Could you check a few things on this model? Use its own coordinates, in mm. A direction names the side the tool comes from. Coordinates: 2 decimals unless noted, no trailing zeros. Loops run counter-clockwise (first coordinate to the right, second up) from the corner with the lowest first, then second, coordinate; pieces in that order, holes last. Notation, with made-up numbers: (76.25, 14.25) - (100.25, 14.25) arc R13 ccw to (100.25, 18.25) - close; hole circle Ø2 at (83, 29.25). An arc over 180 degrees is marked (long way). One line per question, with ' | ' between items. Start each with the question number.
1. I want a section at B-B, the plane z = 3. Count the separate pieces of the cut face and the enclosed holes in it, then the cut area to 3 significant figures.
2. I want a section at A-A, the plane x = 246.5. Write out the boundary of the cut face in (y, z).
3. We'd pull the mould along Y, two halves only. Please class faces 1 (the flat face through (247, 422, 0)), 2 (the flat face through (265.41, 446.46, 3.7)), 3 (the cylindrical face through (303.067, 434.436, 3.698)), 4 (the flat face through (231.455, 384.982, 3.698)): pulls with the +Y half, pulls with the -Y half, needs draft (parallel to the pull), parting line crosses it, or undercut.
4. Please list where these lines run through material, in increasing order: L1, parallel to Y at x = 241.5, z = 1.25; L2, parallel to Y at x = 276.5, z = 6; L3, parallel to X at y = 426.5, z = 3.25. Write a range as [from, to].
5. I'm going to push flat-ended pins straight in: P1, Ø4, axis at y = 408.5, z = 6, coming from the -X side; P2, Ø4, axis at x = 204.5, y = 400, coming from the +Z side; P3, Ø2, axis at y = 389.5, z = 4.5, coming from the -X side; P4, Ø3, axis at x = 252.5, z = 4, coming from the -Y side. Where does each tip first touch, or does it pass through?
6. Which directions (+Z, -Z, +X, -X, +Y, -Y) give clear straight access to the entire face, cutting with the end or side of a thin tool? Please do faces 5 (the cylindrical face through (279.122, 439.862, 3.698)), 6 (the flat face through (203.159, 445.655, 3.698)).
from build123d import *

# Parameters (mm, degrees)
SKETCH1_R           = 13.83528528
SKETCH1_R_2         = 7.213103978
SKETCH1_R_3         = 7.235591107
SKETCH1_R_4         = 7.205059389
SKETCH1_R_5         = 3.002887994
SKETCH1_R_6         = 3.006464833
SKETCH1_R_7         = 3.009410698
SKETCH1_R_8         = 3.002883417
SKETCH1_R_9         = 3.011320737
BOSS_EXTRUDE3_DEPTH = 10
SCALE6_SCALE        = 0.75


with BuildPart() as part:
    # Sketch1 → Boss-Extrude3 (new body)
    with BuildSketch(Plane.XY):
        with BuildLine():
            Line((388.937137401, 591.801924948), (317.8384, 598.8518))
            Line((317.8384, 598.8518), (286.3759, 593.1514))
            Line((286.3759, 593.1514), (254.9413, 595.2929))
            add(Edge.make_bspline(
                [(254.9413, 595.2929), (249.749, 589.6403), (247.5763, 576.1381), (246.6964, 565.0014)],
                knots=[0.333333333, 0.333333333, 0.333333333, 0.333333333, 0.375, 0.375, 0.375, 0.375], degree=3))
            add(Edge.make_bspline(
                [(246.6964, 565.0014), (246.2536, 559.3969), (253.8266, 545.9237), (260.2361, 536.2788)],
                knots=[0.375, 0.375, 0.375, 0.375, 0.416666667, 0.416666667, 0.416666667, 0.416666667], degree=3))
            add(Edge.make_bspline(
                [(260.2361, 536.2788), (261.9315, 533.7276), (265.3965, 528.2241), (269.3831, 526.0001)],
                knots=[0.416666667, 0.416666667, 0.416666667, 0.416666667, 0.458333333, 0.458333333, 0.458333333, 0.458333333], degree=3))
            add(Edge.make_bspline(
                [(269.3831, 526.0001), (274.7125, 523.027), (280.9349, 523.6791), (284.7215, 523.5997)],
                knots=[0.458333333, 0.458333333, 0.458333333, 0.458333333, 0.5, 0.5, 0.5, 0.5], degree=3))
            Line((284.7215, 523.5997), (294.3118, 523.3986))
            add(Edge.make_bspline(
                [(294.3118, 523.3986), (298.656, 523.1896), (301.8697, 521.53), (304.1649, 518.6915)],
                knots=[0.541666667, 0.541666667, 0.541666667, 0.541666667, 0.583333333, 0.583333333, 0.583333333, 0.583333333], degree=3))
            Line((304.1649, 518.6915), (313.1736, 507.7735))
            add(Edge.make_bspline(
                [(313.1736, 507.7735), (316.1604, 504.7059), (319.8516, 502.9821), (324.4499, 502.9891)],
                knots=[0.625, 0.625, 0.625, 0.625, 0.666666667, 0.666666667, 0.666666667, 0.666666667], degree=3))
            Line((324.4499, 502.9891), (362.1482, 502.591))
            add(Edge.make_bspline(
                [(362.1482, 502.591), (370.3987, 506.5747), (383.2456, 509.8601), (391.8953, 515.4769)],
                knots=[0.708333333, 0.708333333, 0.708333333, 0.708333333, 0.75, 0.75, 0.75, 0.75], degree=3))
            add(Edge.make_bspline(
                [(391.8953, 515.4769), (396.6269, 518.5494), (403.2187, 519.6191), (399.5807, 526.7157)],
                knots=[0.75, 0.75, 0.75, 0.75, 0.791666667, 0.791666667, 0.791666667, 0.791666667], degree=3))
            add(Edge.make_bspline(
                [(399.5807, 526.7157), (397.6964, 530.3909), (395.5139, 533.4064), (388.7679, 530.7766)],
                knots=[0.791666667, 0.791666667, 0.791666667, 0.791666667, 0.833333333, 0.833333333, 0.833333333, 0.833333333], degree=3))
            ThreePointArc((388.7679, 530.7766), (356.972685935, 558.005631546), (397.461737401, 568.635424948))
            add(Edge.make_bspline(
                [(397.461737401, 568.635424948), (400.930937401, 564.911724948), (406.485637401, 566.174424948), (409.760237401, 568.677624948)],
                knots=[0.041666667, 0.041666667, 0.041666667, 0.041666667, 0.083333333, 0.083333333, 0.083333333, 0.083333333], degree=3))
            add(Edge.make_bspline(
                [(409.760237401, 568.677624948), (413.064537401, 571.203624948), (414.760537401, 574.392624948), (410.538737401, 579.771624948)],
                knots=[0.083333333, 0.083333333, 0.083333333, 0.083333333, 0.125, 0.125, 0.125, 0.125], degree=3))
            add(Edge.make_bspline(
                [(410.538737401, 579.771624948), (405.594037401, 586.071924948), (398.916537401, 589.707824948), (390.702437401, 591.546424948)],
                knots=[0.125, 0.125, 0.125, 0.125, 0.166666667, 0.166666667, 0.166666667, 0.166666667], degree=3))
            add(Edge.make_bspline(
                [(390.702437401, 591.546424948), (390.170237401, 591.665524948), (389.498937401, 591.746824948), (388.937137401, 591.801924948)],
                knots=[0.166666667, 0.166666667, 0.166666667, 0.166666667, 0.208333333, 0.208333333, 0.208333333, 0.208333333], degree=3))
        make_face()
        with Locations((278.423738523, 540.940981928)):
            Circle(SKETCH1_R, mode=Mode.SUBTRACT)
        with Locations((319.240426613, 548.839403542)):
            Circle(SKETCH1_R_2, mode=Mode.SUBTRACT)
        with Locations((328.512486768, 515.283376314)):
            Circle(SKETCH1_R_3, mode=Mode.SUBTRACT)
        with Locations((323.793948601, 581.881607046)):
            Circle(SKETCH1_R_4, mode=Mode.SUBTRACT)
        with Locations((402.475445199, 576.716414423)):
            Circle(SKETCH1_R_5, mode=Mode.SUBTRACT)
        with Locations((370.54631834, 583.947774508)):
            Circle(SKETCH1_R_6, mode=Mode.SUBTRACT)
        with Locations((348.329436617, 559.905288749)):
            Circle(SKETCH1_R_7, mode=Mode.SUBTRACT)
        with Locations((358.027351347, 528.638383691)):
            Circle(SKETCH1_R_8, mode=Mode.SUBTRACT)
        with Locations((389.953559171, 521.398342198)):
            Circle(SKETCH1_R_9, mode=Mode.SUBTRACT)
    extrude(amount=BOSS_EXTRUDE3_DEPTH)


with BuildPart() as part_1:
    # Scale6: scaled about (0, 0, 0)
    add(part.part.scale(SCALE6_SCALE))


solid = part_1.part
Results are:
1) separate pieces: 1 | enclosed holes: 9 | area: 5,220 mm2
2) outline: (377.21, 0) - (381.04, 0) - (381.04, 7.5) - (377.21, 7.5) - close; (391.89, 0) - (432.43, 0) - (432.43, 7.5) - (391.89, 7.5) - close; (440.39, 0) - (448.33, 0) - (448.33, 7.5) - (440.39, 7.5) - close
3) face 1: needs draft | face 2: pulls with the +Y half | face 3: undercut | face 4: pulls with the -Y half
4) L1: y = [377.37, 384.1], [388.83, 406.63], [416.63, 431.18], [441.64, 448.83] | L2: y = [379.01, 398.99], [430.09, 436.2], [439.72, 445.36] | L3: x = [185.27, 271.93], [298.07, 307.31]
5) P1: stops at x = 190.09 | P2: passes through | P3: stops at x = 226.63 | P4: stops at y = 377.13
6) face 5: +Z, -Z | face 6: +Z, -Z, +Y
